Autodesk Inventor part; units mm, degrees
ref_plane "YZ Plane" through (0, 0, 0) normal (1, 0, 0) x (0, 1, 0)
ref_plane "XZ Plane" through (0, 0, 0) normal (0, 1, 0) x (-1, 0, 0)
ref_plane "XY Plane" through (0, 0, 0) normal (0, 0, 1) x (1, 0, 0)
sketch "Sketch1" plane through (0, 0, 0) normal (0, 1, 0) x (-1, 0, 0)
  line L0 (0, 17.4625) -> (0, 1.5875)
  line L1 (1.5875, 0) -> (17.4625, 0)
  line L2 (17.4625, 0) -> (17.4625, -1.5875)
  line L3 (17.4625, -1.5875) -> (-1.5875, -1.5875)
  line L4 (-1.5875, -1.5875) -> (-1.5875, 17.4625)
  line L5 (-1.5875, 17.4625) -> (0, 17.4625)
  arc A0 (0, 1.5875) -> (1.5875, 0) centre (1.5875, 1.5875) ccw
  point P0 (0, 0)
  dimension "d0" = 1.5875
  dimension "d1" = 19.05
  dimension "d2" = 1.5875
extrude "Extrusion1" add sketch "Sketch1" along normal blind 323.85
properties part number "Short Wall Cross" material "Aluminum 6061"
Design review of the part built by this model. Coordinates are the model's own, in mm. A direction names the side the tool comes from. Give positions to 0.01 mm unless a question says otherwise; leave off trailing zeros. Order: outer loops, then holes, each group sorted by start corner. A loop starts at its lowest first (then second) coordinate and runs counter-clockwise, first axis right, second up. Notation, with made-up numbers: (49.5, 74) - (65.5, 74) arc R15 ccw to (65.5, 89) - close; hole circle Ø7 at (60, 37). An arc over 180 degrees is marked (long way). Use CSV: the item, a comma, the result in double quotes. Start each with the question number.
Q1. Take a section at A-A (y = 263.5). State the section outline as (x, z) points (1 decimal), and give its area (3 significant figures).
Q2. Take a section at C-C (x = -12). State the section outline as (y, z) points.
Q3. Machinability: for faces 1 (the face through (-9, 160, 0)), 2 (the face through (-3.7, 323.85, -0.5)), which of the approach directions +Z, -Z, +X, -X, +Y, -Y give a long, thin tool a straight path to every point of the face, cutting with its end or side? Answer none if there is none.
Q4. For P1, Ø5, axis at x = -6.5, y = 122, coming from the +Z side; P2, Ø2, axis at y = 162, z = 7.5, coming from the -X side; P3, Ø6, axis at x = -1.5, y = 265.5, coming from the +Z side; P4, Ø10, axis at x = -6.5, z = 6, coming from the -Y side, all flat-tipped, find the tip position at first contact; note any pin that passes through.
Q5. Draft analysis for pull direction X (two halves, no side actions). For faces 3 (the face through (-8, 160, -1.588)), 4 (the face through (1.588, 160, 8)), 5 (the face through (0, 160, 10)), state which applies: pulls with the +X half, pulls with the -X half, needs draft (parallel to the pull), parting line crosses it, or undercut.
Q6. For line 1 (X direction, y = 152, z = 12.75); line 2 (Z direction, x = -12.25, y = 256.5); line 3 (Z direction, x = -0.5, y = 51), list the stretches that pass through material, from the lowest coordinate up.
Q7. Take a section at B-B (z = 12.5). State the section outline as (x, y) points.
Calculated:
1,outline,"(-17.5, -1.6) - (1.6, -1.6) - (1.6, 17.5) - (0, 17.5) - (0, 1.6) arc R1.6 cw to (-1.6, 0) - (-17.5, 0) - close"
1,area,"58.5 mm²"
2,outline,"(0, -1.59) - (323.85, -1.59) - (323.85, 0) - (0, 0) - close"
3,face 1,"+Z, -X, +Y, -Y"
3,face 2,"+Z, -Z, +X, -X, +Y"
4,P1,"stops at z = 0"
4,P2,"stops at x = 0"
4,P3,"stops at z = 17.46"
4,P4,"passes through"
5,face 3,"needs draft"
5,face 4,"pulls with the +X half"
5,face 5,"pulls with the -X half"
6,line 1,"x = 0 to 1.59"
6,line 2,"z = -1.59 to 0"
6,line 3,"z = -1.59 to 0.43"
7,outline,"(0, 0) - (1.59, 0) - (1.59, 323.85) - (0, 323.85) - close"
